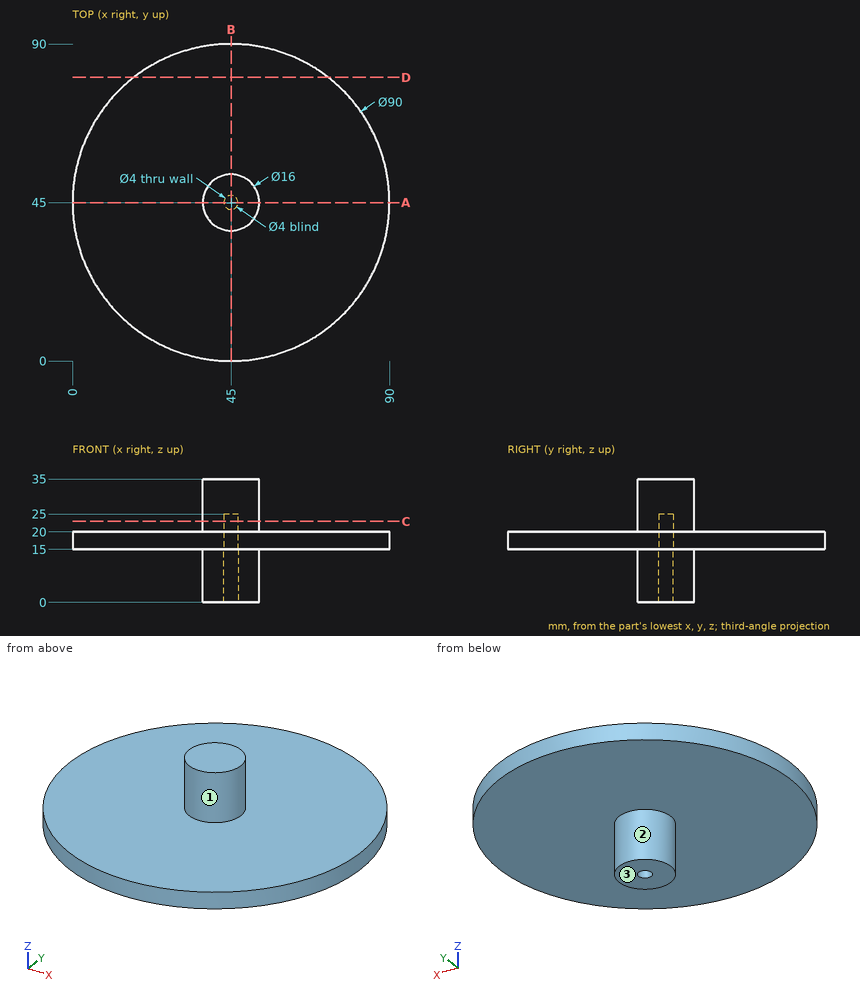
Study the drawing (mm; zero at the part's minimum x, y, z) and answer. A direction names the side the tool comes from. Give positions to 0.01 mm unless a question says otherwise; leave off trailing zeros. Loops run counter-clockwise (first coordinate to the right, second up) from the corner with the lowest first, then second, coordinate; pieces in that order, holes last. Notation, with made-up numbers: (-38.75, -21.5) - (3.25, -21.5) arc R31 cw to (3.25, 5.5) - close; hole circle Ø7 at (-2.75, 76). An arc over 180 degrees is marked (long way). Return JSON: item names as keys, results as strings. Group by question number.
1. Given pin 1 Ø12 at (x, z) = (73.5, 27.5) entering from +Y; pin 2 Ø4 at (x, y) = (48.5, 76.5) entering from -Z; pin 3 Ø2 at (x, y) = (25, 11.5) entering from +Z; pin 4 Ø1.5 at (x, z) = (49, 11) entering from +Y, each flat-ended and moving along its own axis, determine where each tip first touches the part or whether it passes through.
2. Find section A-A (y = 45). Write down the section's boundary in (x, z).
3. Find section D-D (y = 80.5). Write down the section's boundary in (x, z), then the cut area to 3 significant figures.
4. Which of the six approach directions +Z, -Z, +X, -X, +Y, -Y give full straight-line access (tool end or side, diameter ignored) to the marked faces 1, 2 and 3?
5. Find section C-C (z = 23). Write down the section's boundary in (x, y), then the cut area to 3 significant figures.
6. Straight lines are drawn through the part: line 1 (Y direction, x = 45, z = 19.25); line 2 (Y direction, x = 45, z = 9.75); line 3 (Z direction, x = 65, y = 24.5). For each, find the intervals that lie inside material, in ascending order. Write a range as [from, to].
Verdict:
{
 "1": {"pin 1": "passes through", "pin 2": "stops at z = 15", "pin 3": "stops at z = 20", "pin 4": "stops at y = 52.31"},
 "2": {"outline": "(0, 15) - (37, 15) - (37, 0) - (43, 0) - (43, 25) - (47, 25) - (47, 0) - (53, 0) - (53, 15) - (90, 15) - (90, 20) - (53, 20) - (53, 35) - (37, 35) - (37, 20) - (0, 20) - close"},
 "3": {"outline": "(17.35, 15) - (72.65, 15) - (72.65, 20) - (17.35, 20) - close", "area": "277 mm^2"},
 "4": {"face 1": "+Z", "face 2": "-Z", "face 3": "-Z, +X, -X, +Y, -Y"},
 "5": {"outline": "circle Ø16 at (45, 45); hole circle Ø4 at (45, 45)", "area": "188 mm^2"},
 "6": {"line 1": "y = [0, 43], [47, 90]", "line 2": "y = [37, 43], [47, 53]", "line 3": "z = [15, 20]"}
}
